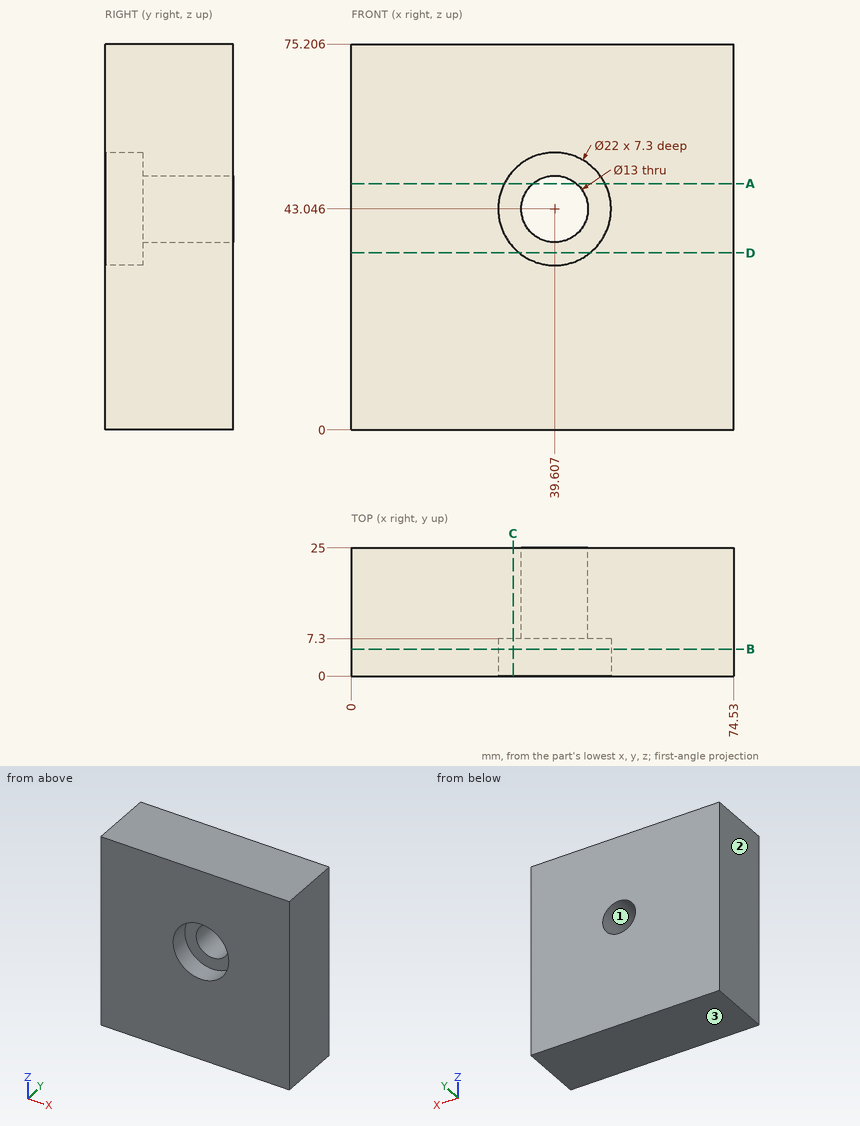
Verification items for this drawing (mm, ordinates from the low corner). Coordinates: 2 decimals unless noted, no trailing zeros. Order: outer loops, then holes, each group sorted by start corner. A loop starts at its lowest first (then second) coordinate and runs counter-clockwise, first axis right, second up. Notation, with made-up numbers: (26.5, 10) - (76.5, 10) arc R29 ccw to (76.5, 45) - close; hole circle Ø9 at (89, 12). An arc over 180 degrees is marked (long way). Use one line per item in the form item = value.
1. Scan lines: line 1 (X direction, y = 1, z = 39.5) (1 decimal); line 2 (Z direction, x = 38.5, y = 2.25); line 3 (X direction, y = 23.5, z = 46). Record each from-to range of solid material in increasing order.
Here are the results:
line_1 = 0 to 29.2, 50 to 74.5
line_2 = 0 to 32.1, 53.99 to 75.21
line_3 = 0 to 33.82, 45.4 to 74.53
2. Draft check along Z on the marked faces 1, 2 and 3. Enter one of: pulls with the +Z half, pulls with the -Z half, needs draft (parallel to the pull), parting line crosses it, or undercut.
Here are the results:
face_1 = undercut
face_2 = needs draft
face_3 = pulls with the -Z half
3. Section check D-D (z = 34.5). Record the boundary of the cut face in (x, y).
Here are the results:
outline = (0, 0) - (32.68, 0) - (32.68, 7.3) - (46.53, 7.3) - (46.53, 0) - (74.53, 0) - (74.53, 25) - (0, 25) - close
4. Section check A-A (z = 48). Record the boundary of the cut face in (x, y) (1 decimal).
Here are the results:
outline = (0, 0) - (29.8, 0) - (29.8, 7.3) - (35.4, 7.3) - (35.4, 25) - (0, 25) - close; (43.8, 7.3) - (49.4, 7.3) - (49.4, 0) - (74.5, 0) - (74.5, 25) - (43.8, 25) - close
5. Section check B-B (y = 5.25). Record the boundary of the cut face in (x, z) (1 decimal).
Here are the results:
outline = (0, 0) - (74.5, 0) - (74.5, 75.2) - (0, 75.2) - close; hole circle Ø22 at (39.6, 43)
6. Gauge pin test, flat ends, axial feed: pin 1 (11.5 mm diameter, centred on x = 39.61, z = 43.05, fed in from -Y); pin 2 (12 mm diameter, centred on x = 59.5, z = 15.5, fed in from -Y); pin 3 (17.5 mm diameter, centred on x = 39.61, z = 43.05, fed in from -Y). Record the tip position at first contact, or that the pin passes through.
Here are the results:
pin_1 = through
pin_2 = 0
pin_3 = 7.3
7. Section check C-C (x = 31.5). Record the boundary of the cut face in (y, z).
Here are the results:
outline = (0, 0) - (25, 0) - (25, 75.21) - (0, 75.21) - (0, 50.48) - (7.3, 50.48) - (7.3, 35.61) - (0, 35.61) - close
